Part model, mm, in its own coordinate system. Face numbers are marked on the shaded views. A direction names the side the tool comes from. Round coordinates to 2 decimals unless told otherwise and drop trailing zeros. Order: outer loops, then holes, each group sorted by start corner. A loop starts at its lowest first (then second) coordinate and runs counter-clockwise, first axis right, second up. Notation, with made-up numbers: (-16, 85.5) - (-12, 85.5) arc R9 cw to (-12, 97.5) - close; hole circle Ø6 at (29.5, 66.25). An arc over 180 degrees is marked (long way). Return JSON: item names as keys, results as strings. Group by question number.
Item 1: Saw through at A-A on z = -3.25. List the corners of the cut face in (x, y).
Item 2: Saw through at C-C on x = -55. List the corners of the cut face in (y, z).
Item 3: Drop flat-ended pins along their axis: pin 1 (19.5 mm diameter, centred on x = 41, y = -6.5, fed in from -Z); pin 2 (1.2 mm diameter, centred on y = 5, z = -7, fed in from +X); pin 3 (4 mm diameter, centred on x = -0.5, y = -20.5, fed in from +Z). Give the stop position or say it passes through.
Item 4: Probe probe 1 along Y at (x, z) = (57, -2.15); probe 2 along X at (y, z) = (28, 2.05); probe 3 along X at (y, z) = (31, 1). List the from-to ranges inside material, lowest first.
Item 5: Tool access for the marked faces 4, 5 and 6: list every direction of +Z, -Z, +X, -X, +Y, -Y with a clear straight run to the whole face (end or side of a thin tool).
Item 6: Two-plate mould, pull along X, no slides. Class the marked faces 1, 2 and 3: released by +X, released by -X, zero draft, split by the parting line, or undercut.
Item 7: Saw through at D-D on x = -1.5. List the corners of the cut face in (y, z).
Item 8: Saw through at B-B on y = -6.5. List the corners of the cut face in (x, z).
```python
from build123d import *

# Parameters (mm, degrees)
F1_DEPTH = 40
F2_R     = 4
F3_DEPTH = 40


with BuildPart() as f1:
    # F0 (on Front) → F1 (new body, symmetric)
    with BuildSketch(Plane.XZ):
        Polygon((-69, 5), (-69, -5), (-30, -5), (-30, -9), (30, -9), (30, -5), (69, -5), (69, 5), (25, 5), (25, 2), (-25, 2), (-25, 5), align=None)
    extrude(amount=F1_DEPTH, both=True)

    # F2 (on Top) → F3 (cut, symmetric)
    with BuildSketch(Plane.XY):
        with BuildLine():
            ThreePointArc((-69, 28), (-65.485281, 36.485281), (-57, 40))
            Line((-57, 40), (-69, 40))
            Line((-69, 40), (-69, 28))
        make_face()
        with BuildLine():
            ThreePointArc((-57, -40), (-65.485281, -36.485281), (-69, -28))
            Line((-69, -28), (-69, -40))
            Line((-69, -40), (-57, -40))
        make_face()
        with BuildLine():
            ThreePointArc((69, -28), (65.485281, -36.485281), (57, -40))
            Line((57, -40), (69, -40))
            Line((69, -40), (69, -28))
        make_face()
        with BuildLine():
            ThreePointArc((57, 40), (65.485281, 36.485281), (69, 28))
            Line((69, 28), (69, 40))
            Line((69, 40), (57, 40))
        make_face()
        with Locations((-57, 28)):
            Circle(F2_R)
        with Locations((57, 28)):
            Circle(F2_R)
        with Locations((57, -28)):
            Circle(F2_R)
        with Locations((-57, -28)):
            Circle(F2_R)
    extrude(amount=F3_DEPTH, both=True, mode=Mode.SUBTRACT)


solid = f1.part
```
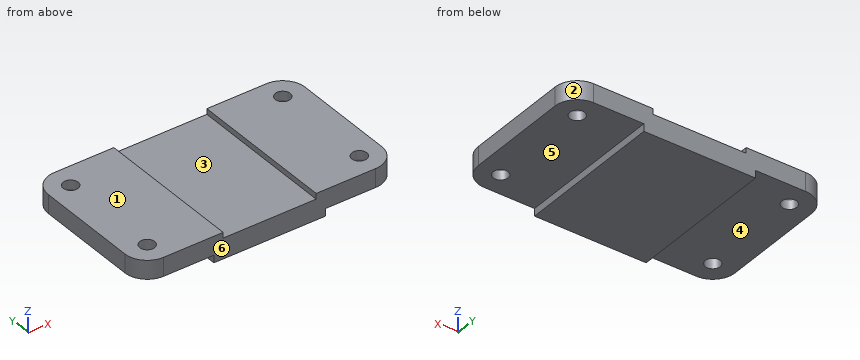
Filled in:
{
 "1": {"outline": "(-69, -28) arc R12 ccw to (-57, -40) - (57, -40) arc R12 ccw to (69, -28) - (69, 28) arc R12 ccw to (57, 40) - (-57, 40) arc R12 ccw to (-69, 28) - close; hole circle Ø8 at (-57, -28); hole circle Ø8 at (-57, 28); hole circle Ø8 at (57, -28); hole circle Ø8 at (57, 28)"},
 "2": {"outline": "(-40, -5) - (-31.46, -5) - (-31.46, 5) - (-40, 5) - close; (-24.54, -5) - (24.54, -5) - (24.54, 5) - (-24.54, 5) - close; (31.46, -5) - (40, -5) - (40, 5) - (31.46, 5) - close"},
 "3": {"pin 1": "stops at z = -5", "pin 2": "stops at x = 30", "pin 3": "stops at z = 2"},
 "4": {"probe 1": "y = -40 to -32, -24 to 24, 32 to 40", "probe 2": "x = -69 to -61, -53 to -25, 25 to 53, 61 to 69", "probe 3": "x = -68.62 to -59.65, -54.35 to 54.35, 59.65 to 68.62"},
 "5": {"face 4": "-Z, -X, +Y, -Y", "face 5": "-Z, +X, +Y, -Y", "face 6": "+Z, -Z, +X, -X, -Y"},
 "6": {"face 1": "zero draft", "face 2": "released by +X", "face 3": "undercut"},
 "7": {"outline": "(-40, -9) - (40, -9) - (40, 2) - (-40, 2) - close"},
 "8": {"outline": "(-69, -5) - (-30, -5) - (-30, -9) - (30, -9) - (30, -5) - (69, -5) - (69, 5) - (25, 5) - (25, 2) - (-25, 2) - (-25, 5) - (-69, 5) - close"}
}
